Design review of the part shown in the three views and the two pictorial views. Dimensions are in mm from the part's minimum x, y and z. Coordinates: 2 decimals unless noted, no trailing zeros. Loops run counter-clockwise (first coordinate to the right, second up) from the corner with the lowest first, then second, coordinate; pieces in that order, holes last. Notation, with made-up numbers: (-10, -22) - (10, -22) arc R23 ccw to (10, -12) - close; hole circle Ø10 at (13.25, 20). An arc over 180 degrees is marked (long way). One line per question, with ' | ' between items.
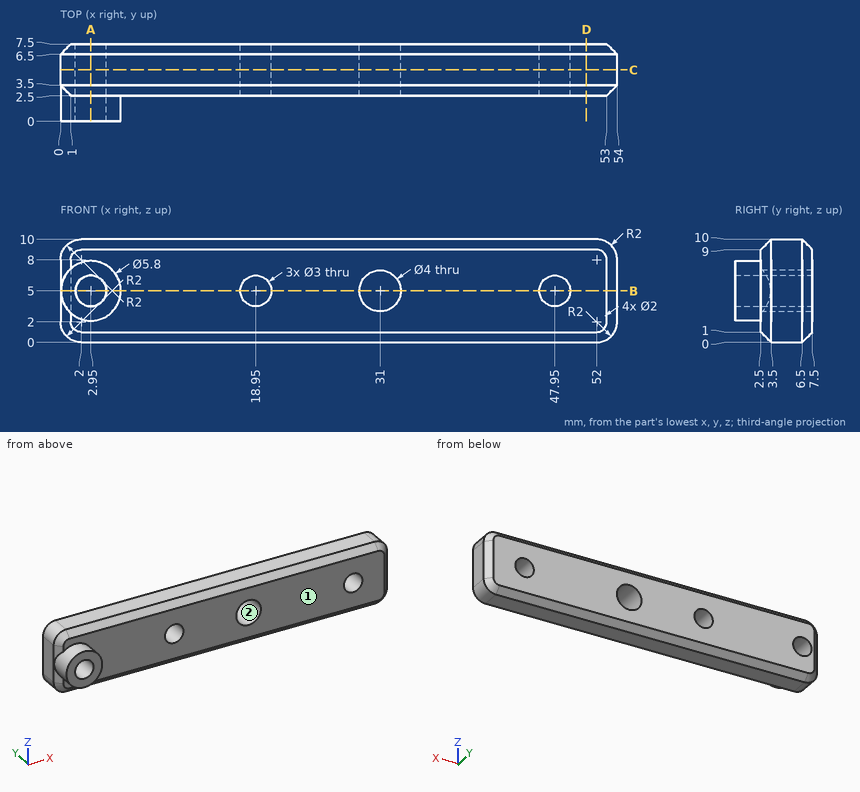
Q1. Draft analysis for pull direction X (two halves, no side actions). For the marked faces 1 and 2, state which applies: +X half, -X half, draft (parallel to the pull), parting line (faces both ways), or undercut.
Returned:
face 1: draft | face 2: undercut
Q2. For pin 1 (1.5 mm diameter, centred on x = 13, z = 8, fed in from -Y); pin 2 (4 mm diameter, centred on x = 47.95, z = 5, fed in from +Y); pin 3 (3.5 mm diameter, centred on x = 31, z = 5, fed in from -Y), all flat-tipped, find the tip position at first contact; note any pin that passes through.
Returned:
pin 1: stops at y = 2.5 | pin 2: stops at y = 7.5 | pin 3: passes through
Q3. To check wall thickness, follow line 1 along X through (y, z) = (6.15, 5); line 2 along Y through (x, z) = (34.5, 8); line 3 along Y through (x, z) = (17.5, 9.5). State the ranges of each line that lie inside material, in increasing order.
Returned:
line 1: x = 0 to 1.45, 4.45 to 17.45, 20.45 to 29, 33 to 46.45, 49.45 to 54 | line 2: y = 2.5 to 7.5 | line 3: y = 3 to 7
Q4. Take a section at B-B (z = 5). Give the boundary of the cut face in (x, y), plus the area to 3 significant figures.
Returned:
outline: (0, 3.5) - (0.05, 3.45) - (0.05, 0) - (1.45, 0) - (1.45, 7.5) - (1, 7.5) - (0, 6.5) - close; (4.45, 0) - (5.85, 0) - (5.85, 2.5) - (17.45, 2.5) - (17.45, 7.5) - (4.45, 7.5) - close; (20.45, 2.5) - (29, 2.5) - (29, 7.5) - (20.45, 7.5) - close; (33, 2.5) - (46.45, 2.5) - (46.45, 7.5) - (33, 7.5) - close; (49.45, 2.5) - (53, 2.5) - (54, 3.5) - (54, 6.5) - (53, 7.5) - (49.45, 7.5) - close | area: 210 mm²
Q5. Take a section at C-C (y = 5). Give the boundary of the cut face in (x, z), plus the area to 3 significant figures.
Returned:
outline: (0, 2) arc R2 ccw to (2, 0) - (52, 0) arc R2 ccw to (54, 2) - (54, 8) arc R2 ccw to (52, 10) - (2, 10) arc R2 ccw to (0, 8) - close; hole circle Ø3 at (2.95, 5); hole circle Ø3 at (18.95, 5); hole circle Ø4 at (31, 5); hole circle Ø3 at (47.95, 5) | area: 503 mm²
Q6. Take a section at D-D (x = 51). Give the boundary of the cut face in (y, z).
Returned:
outline: (2.5, 1) - (3.5, 0) - (6.5, 0) - (7.5, 1) - (7.5, 9) - (6.5, 10) - (3.5, 10) - (2.5, 9) - close
Q7. Take a section at A-A (x = 2.95). Give the boundary of the cut face in (y, z), plus the area to 3 significant figures.
Returned:
outline: (0, 2.1) - (2.5, 2.1) - (2.5, 1) - (3.5, 0) - (6.5, 0) - (7.5, 1) - (7.5, 3.5) - (0, 3.5) - close; (0, 6.5) - (7.5, 6.5) - (7.5, 9) - (6.5, 10) - (3.5, 10) - (2.5, 9) - (2.5, 7.9) - (0, 7.9) - close | area: 40.0 mm²
